Source: CAD feature listing. Evaluate the final solid. Frame: model axes, mm. Round coordinates to 2 decimals unless told otherwise and drop trailing zeros. Write each loop counter-clockwise with the first axis right and the second up, starting at its lowest first coordinate (ties: lowest second). Pieces come first, ordered by that corner, then holes.
from build123d import *

# Parameters (mm, degrees)
SKETCH1_W           = 70
SKETCH1_H           = 30
SKETCH1_R           = 0.6
BOSS_EXTRUDE2_DEPTH = 10
BOSS_EXTRUDE3_DEPTH = 2


with BuildPart() as part:
    # Sketch1 → Boss-Extrude2 (new body)
    with BuildSketch(Plane.XY):
        with Locations((35, 15)):
            Rectangle(SKETCH1_W, SKETCH1_H)
        with Locations((22.55, 15)):
            Circle(SKETCH1_R, mode=Mode.SUBTRACT)
        with Locations((47.45, 15)):
            Circle(SKETCH1_R, mode=Mode.SUBTRACT)
        with BuildLine():
            Line((210, 30), (70, 30))
            Line((70, 30), (70, 0))
            Line((70, 0), (210, 0))
            Line((210, 0), (210, 3.95))
            ThreePointArc((210, 3.95), (198.95, 15), (210, 26.05))
            Line((210, 26.05), (210, 30))
        make_face()
        with BuildLine():
            Line((230, 30), (210, 30))
            Line((210, 30), (210, 26.05))
            ThreePointArc((210, 26.05), (217.813529932, 22.813529932), (221.05, 15))
            ThreePointArc((221.05, 15), (217.813529932, 7.186470068), (210, 3.95))
            Line((210, 3.95), (210, 0))
            Line((210, 0), (230, 0))
            Line((230, 0), (230, 30))
        make_face()
    extrude(amount=BOSS_EXTRUDE2_DEPTH)

    # Sketch1_6 → Boss-Extrude3 (add)
    with BuildSketch(Plane.XY):
        with BuildLine():
            ThreePointArc((221.05, 15), (217.813529932, 22.813529932), (210, 26.05))
            Line((210, 26.05), (210, 22.5))
            ThreePointArc((210, 22.5), (215.303300859, 20.303300859), (217.5, 15))
            ThreePointArc((217.5, 15), (215.303300859, 9.696699141), (210, 7.5))
            Line((210, 7.5), (210, 3.95))
            ThreePointArc((210, 3.95), (217.813529932, 7.186470068), (221.05, 15))
        make_face()
        with BuildLine():
            Line((210, 22.5), (210, 26.05))
            ThreePointArc((210, 26.05), (198.95, 15), (210, 3.95))
            Line((210, 3.95), (210, 7.5))
            ThreePointArc((210, 7.5), (202.5, 15), (210, 22.5))
        make_face()
    extrude(amount=BOSS_EXTRUDE3_DEPTH)


solid = part.part
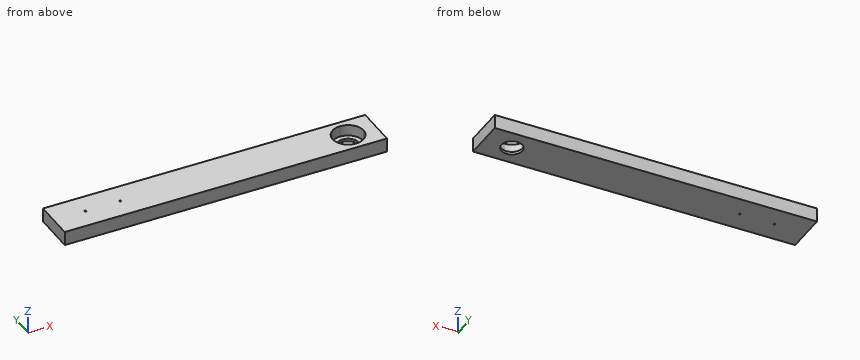
1) Material intervals for line 1 (Y direction, x = 22.55, z = 4.25); line 2 (X direction, y = 14, z = 6.5); line 3 (X direction, y = 17.75, z = 9.25), sorted ascending.
Taken from the geometry:
line 1: y = 0 to 14.4, 15.6 to 30
line 2: x = 0 to 199, 221 to 230
line 3: x = 0 to 199.3, 220.7 to 230
2) Contact query for a flat-ended pin moving along its axis: P1, Ø1, axis at x = 47.45, y = 15, coming from the -Z side. Output: stop coordinate, or through.
Taken from the geometry:
P1: passes through
3) Section query B-B on x = 212.5. Return the cut outline in (y, z).
Taken from the geometry:
outline: (0, 0) - (7.93, 0) - (7.93, 2) - (4.24, 2) - (4.24, 10) - (0, 10) - close; (22.07, 0) - (30, 0) - (30, 10) - (25.76, 10) - (25.76, 2) - (22.07, 2) - close
4) Section query A-A on z = 5. Return the cut outline in (x, y), then the cut area to 3 significant figures.
Taken from the geometry:
outline: (0, 0) - (230, 0) - (230, 30) - (0, 30) - close; hole circle Ø1.2 at (22.55, 15); hole circle Ø1.2 at (47.45, 15); hole circle Ø22.1 at (210, 15)
area: 6,510 mm2
